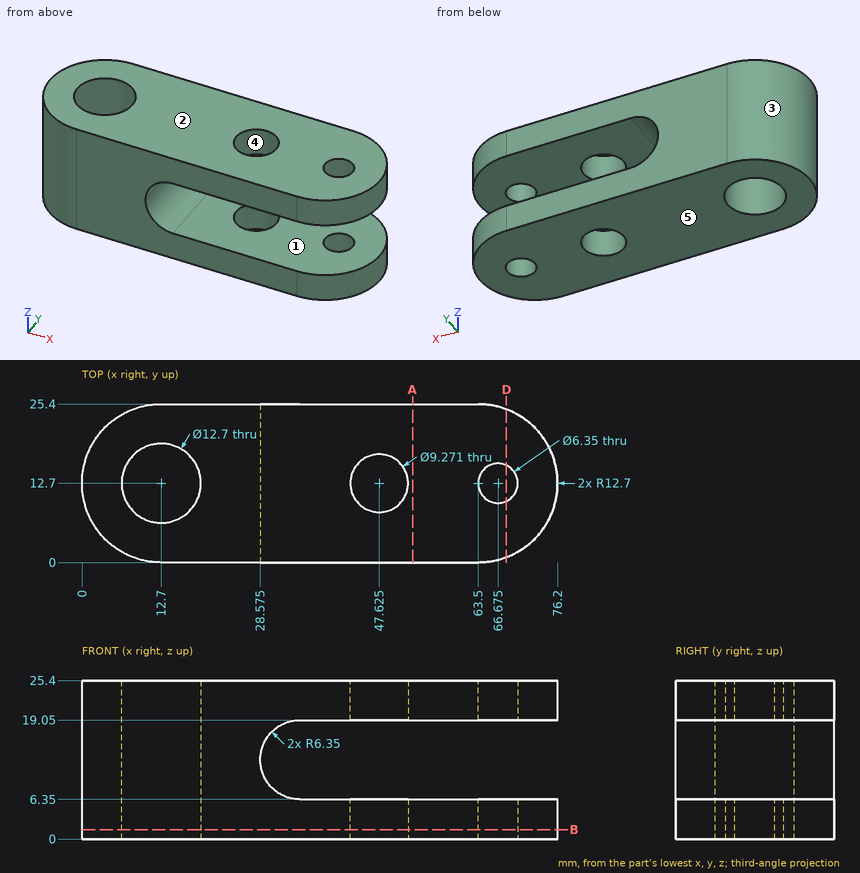
The figure shows three views and two pictorial views of one solid part (mm, origin at its lowest corner). Answer the questions. A direction names the side the tool comes from. Coordinates: 2 decimals unless noted, no trailing zeros. Loops run counter-clockwise (first coordinate to the right, second up) from the corner with the lowest first, then second, coordinate; pieces in that order, holes last. Notation, with made-up numbers: (44.5, 7.25) -> (87.5, 7.25) arc R14 ccw to (87.5, 17.25) -> close; hole circle Ø5 at (63.25, 42). An arc over 180 degrees is marked (long way). Return JSON: item names as keys, results as strings. Group by question number.
(1) Find the intervals of material crossed by probe 1 along Z at (x, y) = (55.5, 24); probe 2 along X at (y, z) = (17.5, 5.5); probe 3 along Y at (x, z) = (49.5, 3.25), in increasing order. Write a range as from..to.
(2) A cutting plane is placed at D-D on x = 68. Write down the section's boundary in (y, z).
(3) A cutting plane is placed at A-A on x = 53. Write down the section's boundary in (y, z).
(4) Determine the mould class of the marked faces 3, 4 and 5 for opening direction Y: released by +Y, released by -Y, zero draft, split by the parting line, or undercut.
(5) Given pin 1 Ø8 at (y, z) = (11, 12.5) entering from +X; pin 2 Ø3 at (y, z) = (11, 13) entering from +X; pin 3 Ø6 at (y, z) = (5, 18.5) entering from -X, each flat-ended and moving along its own axis, determine where each tip first touches the part or whether it passes through.
(6) Which of the six approach directions +Z, -Z, +X, -X, +Y, -Y give full straight-line access (tool end or side, diameter ignored) to the marked faces 1 and 2?
(7) A cutting plane is placed at B-B on z = 1.5. Count the separate pieces of the cut face and the enclosed holes in it, and give its area (3 significant figures).
The answers:
{
 "1": {"probe 1": "z = 0..6.35, 19.05..25.4", "probe 2": "x = 0.94..8.54, 16.86..75.26", "probe 3": "y = 0..8.46, 16.94..25.4"},
 "2": {"outline": "(0.82, 0) -> (9.81, 0) -> (9.81, 6.35) -> (0.82, 6.35) -> close; (0.82, 19.05) -> (9.81, 19.05) -> (9.81, 25.4) -> (0.82, 25.4) -> close; (15.59, 0) -> (24.58, 0) -> (24.58, 6.35) -> (15.59, 6.35) -> close; (15.59, 19.05) -> (24.58, 19.05) -> (24.58, 25.4) -> (15.59, 25.4) -> close"},
 "3": {"outline": "(0, 0) -> (25.4, 0) -> (25.4, 6.35) -> (0, 6.35) -> close; (0, 19.05) -> (25.4, 19.05) -> (25.4, 25.4) -> (0, 25.4) -> close"},
 "4": {"face 3": "split by the parting line", "face 4": "undercut", "face 5": "zero draft"},
 "5": {"pin 1": "stops at x = 30.16", "pin 2": "stops at x = 28.84", "pin 3": "stops at x = 0.9"},
 "6": {"face 1": "+X, +Y, -Y", "face 2": "+Z, +X, -X, +Y, -Y"},
 "7": {"separate pieces": "1", "enclosed holes": "3", "area": "1,570 mm^2"}
}
